Geometry: final body of the model. Coordinates: model frame, mm. Face numbers are marked on the shaded views. Give positions to 0.01 mm unless a question says otherwise; leave off trailing zeros. Write each loop counter-clockwise with the first axis right and the second up, starting at its lowest first coordinate (ties: lowest second). Pieces come first, ordered by that corner, then holes. Notation, with made-up numbers: M 80,47.5 L 102,47.5 A24 cw 102,57.5 Z; hole C 52.25,72 d7. An arc over 180 degrees is marked long. Answer as a JSON object with one key per item and string values.
from build123d import *

# Parameters (mm, degrees)
SKETCH1_W                   = 80
SKETCH1_H                   = 60
BOSS_EXTRUDE1_DEPTH         = 2
SKETCH2_W                   = 3
SKETCH2_H                   = 20
BOSS_EXTRUDE2_DEPTH         = 20
CUT_EXTRUDE1_REACH          = 71.327
SKETCH3_R                   = 3.1
FILLET1_RADIUS              = 10
FILLET1_LENGTH              = 3
CUT_EXTRUDE2_REACH          = 73.877
FILLET1_OF_MIRROR1_2_RADIUS = 10
FILLET1_OF_MIRROR1_2_LENGTH = 3
SKETCH5_W                   = 5
SKETCH5_H                   = 10
BOSS_EXTRUDE3_DEPTH         = 3


with BuildPart() as part:
    # Sketch1 → Boss-Extrude1 (new body)
    with BuildSketch(Plane(origin=(0, 0, 0), x_dir=(1, 0, 0), z_dir=(0, 1, 0))):
        Rectangle(SKETCH1_W, SKETCH1_H)
    extrude(amount=BOSS_EXTRUDE1_DEPTH)

    # Sketch2 → Boss-Extrude2 (add)
    with BuildSketch(Plane(origin=(0, 2, 0), x_dir=(1, 0, 0), z_dir=(0, 1, 0))):
        with Locations((-20, 0)):
            Rectangle(SKETCH2_W, SKETCH2_H)
    boss_extrude2 = extrude(amount=BOSS_EXTRUDE2_DEPTH)

    # Sketch3 → Cut-Extrude1 (cut, up to next)
    with BuildSketch(Plane(origin=(-18.5, 0, 0), x_dir=(0, 0, -1), z_dir=(1, 0, 0)), mode=Mode.PRIVATE) as cut_extrude1_sk1:
        with Locations((0, 14)):
            Circle(SKETCH3_R)
    cut_extrude1_tool1 = extrude(cut_extrude1_sk1.sketch, amount=-CUT_EXTRUDE1_REACH, mode=Mode.PRIVATE) & part.part
    cut_extrude1 = cut_extrude1_tool1.solids().sort_by_distance((-18.5, 14, 0))[0]
    add(cut_extrude1, mode=Mode.SUBTRACT)

    # Fillet1: full round fillet: the end face becomes a half cylinder, R = half its width
    fillet1_face = Plane((-20, 22, 0), x_dir=(-1, 0, 0), z_dir=(0, 1, 0))  # on the end face: x along it, z out of the body
    fillet1_slab = fillet1_face.offset(-FILLET1_RADIUS / 2) * Box(FILLET1_LENGTH, 2 * FILLET1_RADIUS, FILLET1_RADIUS, mode=Mode.PRIVATE)  # the body's end, R deep
    fillet1_round = Plane((-20, 12, 0), x_dir=(0, 1, 0), z_dir=(-1, 0, 0)) * Cylinder(FILLET1_RADIUS, FILLET1_LENGTH, mode=Mode.PRIVATE)  # its axis R under the face
    add(fillet1_slab - fillet1_round, mode=Mode.SUBTRACT)

    # Sketch4 → Cut-Extrude2 (cut, up to next)
    with BuildSketch(Plane.ZY.offset(21.5), mode=Mode.PRIVATE) as cut_extrude2_sk1:
        Polygon((0, 10.9), (5, 23.9), (-5, 23.9), align=None)
    cut_extrude2_tool1 = extrude(cut_extrude2_sk1.sketch, amount=-CUT_EXTRUDE2_REACH, mode=Mode.PRIVATE) & part.part
    cut_extrude2 = cut_extrude2_tool1.solids().sort_by_distance((-21.5, 19.566667, 0))[0]
    add(cut_extrude2, mode=Mode.SUBTRACT)

    # Mirror1: Boss-Extrude2, Cut-Extrude1, Cut-Extrude2 across plane
    add(boss_extrude2.mirror(Plane(origin=(0, 0, 0), x_dir=(0, 0, 1), z_dir=(1, 0, 0))))
    add(cut_extrude1.mirror(Plane(origin=(0, 0, 0), x_dir=(0, 0, 1), z_dir=(1, 0, 0))), mode=Mode.SUBTRACT)
    add(cut_extrude2.mirror(Plane(origin=(0, 0, 0), x_dir=(0, 0, 1), z_dir=(1, 0, 0))), mode=Mode.SUBTRACT)

    # Fillet1 of Mirror1 2: full round fillet: the end face becomes a half cylinder, R = half its width
    fillet1_of_mirror1_2_face = Plane((20, 22, 0), x_dir=(1, 0, 0), z_dir=(0, 1, 0))  # on the end face: x along it, z out of the body
    fillet1_of_mirror1_2_slab = fillet1_of_mirror1_2_face.offset(-FILLET1_OF_MIRROR1_2_RADIUS / 2) * Box(FILLET1_OF_MIRROR1_2_LENGTH, 2 * FILLET1_OF_MIRROR1_2_RADIUS, FILLET1_OF_MIRROR1_2_RADIUS, mode=Mode.PRIVATE)  # the body's end, R deep
    fillet1_of_mirror1_2_round = Plane((20, 12, 0), x_dir=(0, 1, 0), z_dir=(1, 0, 0)) * Cylinder(FILLET1_OF_MIRROR1_2_RADIUS, FILLET1_OF_MIRROR1_2_LENGTH, mode=Mode.PRIVATE)  # its axis R under the face
    add(fillet1_of_mirror1_2_slab - fillet1_of_mirror1_2_round, mode=Mode.SUBTRACT)

    # Sketch5 → Boss-Extrude3 (add)
    with BuildSketch(Plane(origin=(0, 2, 0), x_dir=(1, 0, 0), z_dir=(0, 1, 0))):
        with Locations((-37.5, 0)):
            Rectangle(SKETCH5_W, SKETCH5_H)
    extrude(amount=BOSS_EXTRUDE3_DEPTH)


solid = part.part
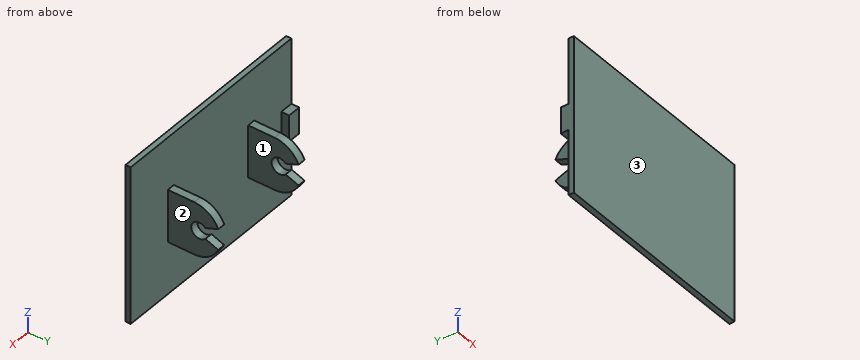
1) Line query: line 1 (X direction, y = 7, z = 3.5); line 2 (Y direction, x = -10, z = 14); line 3 (Z direction, x = -19.2, y = 14). Output: solid intervals per line, ascending. Write a range as from..to.
Geometry check:
{"line 1": "x = -21.5..-18.5, 18.5..21.5", "line 2": "y = 0..2", "line 3": "z = -9.8..-3.1, 3.1..9.8"}
2) Cut plane B-B on y = 14. Return loops of the section in (x, z).
Geometry check:
{"outline": "M -21.5,-9.8 L -18.5,-9.8 L -18.5,-3.1 L -21.5,-3.1 Z; M -21.5,3.1 L -18.5,3.1 L -18.5,9.8 L -21.5,9.8 Z; M 18.5,-9.8 L 21.5,-9.8 L 21.5,-3.1 L 18.5,-3.1 Z; M 18.5,3.1 L 21.5,3.1 L 21.5,9.8 L 18.5,9.8 Z"}
3) Contact query for flat-ended pins moving along their axis: P1, Ø2.5, axis at x = -20.5, y = 5, coming from the -Z side; P2, Ø12, axis at x = 22, z = -16.5, coming from the +Y side; P3, Ø7, axis at y = 14, z = 0, coming from the -X side; P4, Ø3.5, axis at y = 3, z = -1.5, coming from the +X side. Output: stop coordinate, or through.
Geometry check:
{"P1": "stops at z = -10", "P2": "stops at y = 2", "P3": "stops at x = -21.5", "P4": "stops at x = 40"}
4) Cut plane D-D on x = -15.5. Return loops of the section in (y, z), and give its area (3 significant figures).
Geometry check:
{"outline": "M 0,-30 L 2,-30 L 2,30 L 0,30 Z", "area": "120 mm2"}
5) Cut plane C-C on z = 7.5. Return loops of the section in (x, y).
Geometry check:
{"outline": "M -40,0 L 40,0 L 40,2 L 21.5,2 L 21.5,18.61 L 18.5,18.61 L 18.5,2 L -18.5,2 L -18.5,18.61 L -21.5,18.61 L -21.5,2 L -40,2 Z"}
6) Pull-direction query (X, two-part tool) for the marked faces 1, 2 and 3; classes: pulls with the +X half, pulls with the -X half, needs draft (parallel to the pull), parting line crosses it, or undercut.
Geometry check:
{"face 1": "undercut", "face 2": "pulls with the +X half", "face 3": "needs draft"}
7) Cut plane A-A on y = 8.5. Return loops of the section in (x, z).
Geometry check:
{"outline": "M -21.5,-10 L -18.5,-10 L -18.5,10 L -21.5,10 Z; M 18.5,-10 L 21.5,-10 L 21.5,10 L 18.5,10 Z"}
